from build123d import *

# Parameters (mm, degrees)
F0_W     = 8.6
F0_H     = 4.1
F0_W_2   = 9.2
F0_H_2   = 11.5
F1_DEPTH = 1.5
F2_D     = 5.2
F2_DEPTH = 2
F2_TIP   = 1.5622376095
F3_D     = 7
F3_DEPTH = 2
F3_TIP   = 2.1030121666
F4_D     = 5.3
F4_DEPTH = 2
F4_TIP   = 1.5922806404


# Not quite as in the source:
# - a feature names something its author has since deleted; it is built from what else it names


with BuildPart() as f1:
    # F0 (on Top) → F1 (new body)
    with BuildSketch(Plane.XY):
        with BuildLine():
            Line((-37.75, -21), (37.75, -21))
            ThreePointArc((37.75, -21), (42.6997474683, -18.9497474683), (44.75, -14))
            Line((44.75, -14), (44.75, 14))
            ThreePointArc((44.75, 14), (42.6997474683, 18.9497474683), (37.75, 21))
            Line((37.75, 21), (-37.75, 21))
            ThreePointArc((-37.75, 21), (-42.6997474683, 18.9497474683), (-44.75, 14))
            Line((-44.75, 14), (-44.75, -14))
            ThreePointArc((-44.75, -14), (-42.6997474683, -18.9497474683), (-37.75, -21))
        make_face()
        with Locations((-5.25, -14.65)):
            Rectangle(F0_W, F0_H, mode=Mode.SUBTRACT)
        with Locations((-19.43, -5.25)):
            Rectangle(F0_W_2, F0_H_2, mode=Mode.SUBTRACT)
    extrude(amount=F1_DEPTH)

    # F2
    with Locations(Plane(origin=(0, 0, 0), x_dir=(1, 0, 0), z_dir=(0, 0, -1))):
        with Locations((18.75, 7), (-28.75, 7)):
            Hole(F2_D / 2, depth=F2_DEPTH)
            with Locations((0, 0, -(F2_DEPTH + F2_TIP / 2))):  # 118° drill point
                Cone(0, F2_D / 2, F2_TIP, mode=Mode.SUBTRACT)

    # F3
    with Locations(Plane(origin=(0, 0, 0), x_dir=(1, 0, 0), z_dir=(0, 0, -1))):
        with Locations((7.55, 7)):
            Hole(F3_D / 2, depth=F3_DEPTH)
            with Locations((0, 0, -(F3_DEPTH + F3_TIP / 2))):  # 118° drill point
                Cone(0, F3_D / 2, F3_TIP, mode=Mode.SUBTRACT)

    # F4
    with Locations(Plane(origin=(0, 0, 0), x_dir=(1, 0, 0), z_dir=(0, 0, -1))):
        with Locations((-30.2482247353, -5.4)):
            Hole(F4_D / 2, depth=F4_DEPTH)
            with Locations((0, 0, -(F4_DEPTH + F4_TIP / 2))):  # 118° drill point
                Cone(0, F4_D / 2, F4_TIP, mode=Mode.SUBTRACT)


solid = f1.part
Read the model definition and answer for the solid it produces. Units are mm, in the model's axes. A direction names the side the tool comes from. Coordinates: 2 decimals unless noted, no trailing zeros. Order: outer loops, then holes, each group sorted by start corner. A loop starts at its lowest first (then second) coordinate and runs counter-clockwise, first axis right, second up. Notation, with made-up numbers: M -12,48.25 L 6,48.25 A26 cw 6,70.25 Z; hole C 37,7 d3. An arc over 180 degrees is marked long. Put each result on its own line as item: value. Start each with the question number.
Item 1: Given pin 1 Ø4.5 at (x, y) = (-28.75, -7) entering from -Z, flat-ended and moving along its own axis, determine where the tip first touches the part or whether it passes through.
Item 2: The mould has two halves that part along X. Classify faces 1 (the face through (42.65, -19, 0.74)), 2 (the face through (-5, -12.6, 1)), 3 (the face through (-1, 0, 1.5)): +X half, -X half, draft (parallel to the pull), parting line (faces both ways), or undercut.
Item 3: Consider probe 1 along Y at (x, z) = (-3, 0.4); probe 2 along Y at (x, z) = (18.75, 0.4); probe 3 along Y at (x, z) = (-28.75, 1). Determine where each line is inside the solid, lowest interval first. Write a range as [from, to].
Item 4: For faces 4 (the face through (1, 21, 1)), 5 (the face through (-19, 0.5, 1)), determine the directions among +Z, -Z, +X, -X, +Y, -Y from which every point of the face is accessible in a straight line to the end or side of a thin tool.
Item 5: Section B-B, the plane y = -7 is taken. Determine the outline of the cut face in (x, z), plus the area to 4 significant figures.
Item 6: Section A-A, the plane x = -17.5 is taken. Determine the outline of the cut face in (y, z).
Item 7: Section D-D, the plane y = 5.4 is taken. Determine the outline of the cut face in (x, z).
Item 8: Section C-C, the plane z = 0.5 is taken. Determine the outline of the cut face in (x, y).
Computed:
1. pin 1: passes through
2. face 1: +X half
2. face 2: undercut
2. face 3: draft
3. probe 1: y = [-21, -16.7], [-12.6, 21]
3. probe 2: y = [-21, -9.6], [-4.4, 21]
3. probe 3: y = [-21, -9.6], [-4.4, 3.21], [7.59, 21]
4. face 4: +Z, -Z, +X, -X, +Y
4. face 5: +Z, -Z
5. outline: M -44.75,0 L -31.35,0 L -31.35,1.5 L -44.75,1.5 Z; M -26.15,0 L -24.03,0 L -24.03,1.5 L -26.15,1.5 Z; M -14.83,0 L 4.05,0 L 4.05,1.5 L -14.83,1.5 Z; M 11.05,0 L 16.15,0 L 16.15,1.5 L 11.05,1.5 Z; M 21.35,0 L 44.75,0 L 44.75,1.5 L 21.35,1.5 Z
5. area: 94.35 mm2
6. outline: M -21,0 L -11,0 L -11,1.5 L -21,1.5 Z; M 0.5,0 L 21,0 L 21,1.5 L 0.5,1.5 Z
7. outline: M -44.75,0 L -32.9,0 L -32.9,1.5 L -44.75,1.5 Z; M -27.6,0 L 44.75,0 L 44.75,1.5 L -27.6,1.5 Z
8. outline: M -44.75,-14 A7 ccw -37.75,-21 L 37.75,-21 A7 ccw 44.75,-14 L 44.75,14 A7 ccw 37.75,21 L -37.75,21 A7 ccw -44.75,14 Z; hole C -30.25,5.4 d5.3; hole C -28.75,-7 d5.2; hole M -24.03,-11 L -14.83,-11 L -14.83,0.5 L -24.03,0.5 Z; hole M -9.55,-16.7 L -0.95,-16.7 L -0.95,-12.6 L -9.55,-12.6 Z; hole C 7.55,-7 d7; hole C 18.75,-7 d5.2
